Verification items for the finished model (mm, model axes). A direction names the side the tool comes from. Round coordinates to 2 decimals unless told otherwise and drop trailing zeros. Order: outer loops, then holes, each group sorted by start corner. A loop starts at its lowest first (then second) coordinate and runs counter-clockwise, first axis right, second up. Notation, with made-up numbers: M -34,-24 L -18,-24 A29 ccw -18,0 Z; hole C -35.5,2.5 d8. An arc over 180 degrees is marked long. Write item = value, one per line. Start each with the question number.
from build123d import *

# Parameters (mm, degrees)
SKICA1_R                = 1
P_IDAT_VYSUNUT_M1_DEPTH = 2


with BuildPart() as part:
    # Skica1 → Přidat vysunutím1 (new body)
    with BuildSketch(Plane.XY):
        with BuildLine():
            Line((0, 0), (0, -1.5))
            ThreePointArc((0, -1.5), (-2.588190451, -1.840741737), (-5, -2.839745962))
            Line((-5, -2.839745962), (-5.75, -1.540707856))
            Line((-5.75, -1.540707856), (-14.552661177, -1.540707856))
            Line((-14.552661177, -1.540707856), (-28.5, -4))
            Line((-28.5, -4), (-31.5, -4))
            Line((-31.5, -4), (-37.17128182, -3))
            Line((-37.17128182, -3), (-47, -3))
            Line((-47, -3), (-47, 0))
            Line((-47, 0), (0, 0))
        make_face()
        with Locations((-30, -2)):
            Circle(SKICA1_R, mode=Mode.SUBTRACT)
    extrude(amount=P_IDAT_VYSUNUT_M1_DEPTH)


solid = part.part
1) Cross-section at B-B, the plane z = 1.7. Enter the section's corners in (x, y), then the cut area to 3 significant figures.
2) Cross-section at D-D, the plane x = -14. Enter the section's corners in (y, z).
3) Scan lines: probe 1 along Y at (x, z) = (-30, 1.55); probe 2 along Y at (x, z) = (-12, 1.3); probe 3 along Y at (x, z) = (-39.5, 0.95). Record each from-to range of solid material in increasing order.
4) Cross-section at A-A, the plane x = -30. Enter the section's corners in (y, z).
5) Release check for a two-part mould opening along X. For faces 1 (the cylindrical face through (-29, -2, 1)), 2 (the flat face through (-42, -3, 1)), 3 (the flat face through (-47, -2, 1)) record: pulls with the +X half, pulls with the -X half, needs draft (parallel to the pull), parting line crosses it, or undercut.
6) Access from +Z, -Z, +X, -X, +Y, -Y to the whole of each face (thin tool, end or side, straight path). Record for faces 4 (the flat face through (-21.429, -2.753, 0.986)), 5 (the flat face through (-28, -2, 2)).
7) Cross-section at C-C, the plane y = -2. Enter the section's corners in (x, z), then the cut area to 3 significant figures.
8) Gauge pin test, flat end, axial feed: P1, Ø1, axis at x = -10, z = 0.5, coming from the -Y side. Record the tip position at first contact, or that the pin passes through.
Geometry results:
q1.outline = M -47,-3 L -37.17,-3 L -31.5,-4 L -28.5,-4 L -14.55,-1.54 L -5.75,-1.54 L -5,-2.84 A10 cw 0,-1.5 L 0,0 L -47,0 Z; hole C -30,-2 d2
q1.area = 122 mm^2
q2.outline = M -1.54,0 L 0,0 L 0,2 L -1.54,2 Z
q3.probe_1 = -4 to -3, -1 to 0
q3.probe_2 = -1.54 to 0
q3.probe_3 = -3 to 0
q4.outline = M -4,0 L -3,0 L -3,2 L -4,2 Z; M -1,0 L 0,0 L 0,2 L -1,2 Z
q5.face_1 = undercut
q5.face_2 = needs draft
q5.face_3 = pulls with the -X half
q6.face_4 = +Z, -Z, -Y
q6.face_5 = +Z, +X, -X, +Y, -Y
q7.outline = M -47,0 L -31,0 L -31,2 L -47,2 Z; M -29,0 L -17.16,0 L -17.16,2 L -29,2 Z; M -5.48,0 L -3.12,0 L -3.12,2 L -5.48,2 Z
q7.area = 60.4 mm^2
q8.P1 = -1.54
